from build123d import *

# Parameters (mm, degrees)
SKETCH1_W           = 4.77
SKETCH1_H           = 4.01
BOSS_EXTRUDE1_DEPTH = 2.41
SKETCH3_W           = 0.495
SKETCH3_H           = 0.495
BOSS_EXTRUDE2_DEPTH = 13


with BuildPart() as part:
    # Sketch1 → Boss-Extrude1 (new body)
    with BuildSketch(Plane(origin=(0, 0, 0), x_dir=(1, 0, 0), z_dir=(0, 1, 0))):
        with Locations((2.385, -2.005)):
            Rectangle(SKETCH1_W, SKETCH1_H)
    extrude(amount=BOSS_EXTRUDE1_DEPTH)

    # Sketch3 → Boss-Extrude2 (add)
    with BuildSketch(Plane.XY.offset(4.01)):
        with Locations((3.655, 1.205)):
            Rectangle(SKETCH3_W, SKETCH3_H)
        with Locations((2.385, 1.205)):
            Rectangle(SKETCH3_W, SKETCH3_H)
        with Locations((1.115, 1.205)):
            Rectangle(SKETCH3_W, SKETCH3_H)
    extrude(amount=BOSS_EXTRUDE2_DEPTH)


solid = part.part
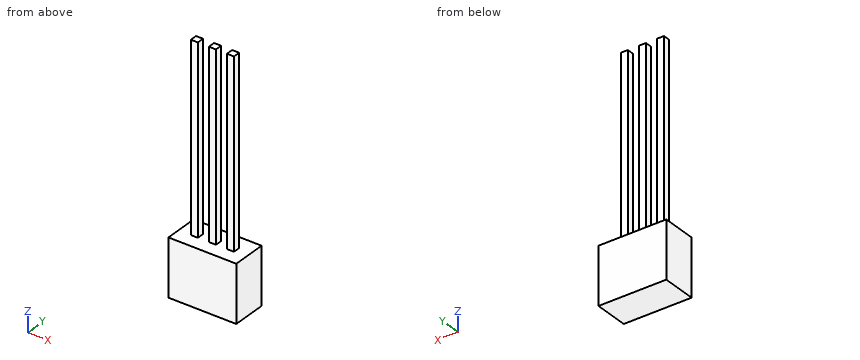
Could you check a few things on this model? Use its own coordinates, in mm. Give positions to 0.01 mm unless a question says otherwise; leave off trailing zeros. Order: outer loops, then holes, each group sorted by start corner. A loop starts at its lowest first (then second) coordinate and runs counter-clockwise, first axis right, second up. Notation, with made-up numbers: (21.5, 27.5) - (71.5, 27.5) arc R18 ccw to (71.5, 52.5) - close; hole circle Ø1 at (44.5, 67). An arc over 180 degrees is marked (long way). One line per question, with ' | ' between items. Start each with the question number.
Item 1: I want a section at C-C on y = 0.25. Write out the boundary of the cut face in (x, z).
Item 2: I want a section at B-B on x = 2.3. Write out the boundary of the cut face in (y, z), then the cut area to 3 significant figures.
Item 3: I need wall thicknesses on probe 1 along X at (y, z) = (1.4, 12); probe 2 along Y at (x, z) = (2.4, 8); probe 3 along Z at (x, y) = (0.9, 2.3). Which ranges of each line are inside material? Lowest first, please. Write a range as [from, to].
Item 4: I want a section at A-A on z = 5. Write out the boundary of the cut face in (x, y), then the cut area to 3 significant figures.
Item 5: I'm going to push flat-ended pins straight in: pin 1 Ø0.5 at (y, z) = (1, 12.5) entering from +X; pin 2 Ø1.5 at (x, z) = (1, 9) entering from +Y. Where does each tip first touch, or does it pass through?
Verdict:
1) outline: (0, 0) - (4.77, 0) - (4.77, 4.01) - (0, 4.01) - close
2) outline: (0, 0) - (2.41, 0) - (2.41, 4.01) - (1.45, 4.01) - (1.45, 17.01) - (0.96, 17.01) - (0.96, 4.01) - (0, 4.01) - close | area: 16.1 mm^2
3) probe 1: [0.87, 1.36], [2.14, 2.63], [3.41, 3.9] | probe 2: [0.96, 1.45] | probe 3: [0, 4.01]
4) outline: (0.87, 0.96) - (1.36, 0.96) - (1.36, 1.45) - (0.87, 1.45) - close; (2.14, 0.96) - (2.63, 0.96) - (2.63, 1.45) - (2.14, 1.45) - close; (3.41, 0.96) - (3.9, 0.96) - (3.9, 1.45) - (3.41, 1.45) - close | area: 0.735 mm^2
5) pin 1: x = 3.9 | pin 2: y = 1.45
